For this review, take the finished solid that the model builds, in its own axes (mm). A direction names the side the tool comes from. Coordinates: 2 decimals unless noted, no trailing zeros. Order: outer loops, then holes, each group sorted by start corner. A loop starts at its lowest first (then second) coordinate and runs counter-clockwise, first axis right, second up.
from build123d import *

# Parameters (mm, degrees)
SKETCH1_W                = 82.55
SKETCH1_H                = 53.086
BOSS_EXTRUDE1_DEPTH      = 4.826
CUT_EXTRUDE1_START       = -88.085249325
CUT_EXTRUDE1_OUTLINE_W   = 4.826
CUT_EXTRUDE1_OUTLINE_H   = 4.826
CUT_EXTRUDE1_DEPTH       = 16.51
CUT_EXTRUDE1_START_2     = -55.065249325
CUT_EXTRUDE1_2_OUTLINE_W = 4.826
CUT_EXTRUDE1_2_OUTLINE_H = 4.826
CUT_EXTRUDE1_2_DEPTH     = 16.51
CUT_EXTRUDE1_START_3     = -22.045249325
CUT_EXTRUDE1_3_OUTLINE_W = 4.826
CUT_EXTRUDE1_3_OUTLINE_H = 4.826
CUT_EXTRUDE1_3_DEPTH     = 16.51
SKETCH3_W                = 4.826
SKETCH3_H                = 12.065
CUT_EXTRUDE2_DEPTH       = 97.443575108
SKETCH4_R                = 12.7
CUT_EXTRUDE3_DEPTH       = 97.443575108
SKETCH5_W                = 4.826
SKETCH5_H                = 12.7
CUT_EXTRUDE4_DEPTH       = 97.443575108


# Read off the part's stored shape, not the designer's step: Cut-Extrude1
with BuildPart() as part:
    # Sketch1 → Boss-Extrude1 (new body)
    with BuildSketch(Plane.XY):
        with Locations((-46.810249325, -12.432142782)):
            Rectangle(SKETCH1_W, SKETCH1_H)
    extrude(amount=BOSS_EXTRUDE1_DEPTH)

    # Cut-Extrude1 outline → Cut-Extrude1 (cut)
    with BuildSketch(Plane.YZ.offset(CUT_EXTRUDE1_START)):
        with Locations((11.697857218, 2.413)):
            Rectangle(CUT_EXTRUDE1_OUTLINE_W, CUT_EXTRUDE1_OUTLINE_H)
    extrude(amount=CUT_EXTRUDE1_DEPTH, mode=Mode.SUBTRACT)

    # Cut-Extrude1 2 outline → Cut-Extrude1 2 (cut)
    with BuildSketch(Plane.YZ.offset(CUT_EXTRUDE1_START_2)):
        with Locations((11.697857218, 2.413)):
            Rectangle(CUT_EXTRUDE1_2_OUTLINE_W, CUT_EXTRUDE1_2_OUTLINE_H)
    extrude(amount=CUT_EXTRUDE1_2_DEPTH, mode=Mode.SUBTRACT)

    # Cut-Extrude1 3 outline → Cut-Extrude1 3 (cut)
    with BuildSketch(Plane.YZ.offset(CUT_EXTRUDE1_START_3)):
        with Locations((11.697857218, 2.413)):
            Rectangle(CUT_EXTRUDE1_3_OUTLINE_W, CUT_EXTRUDE1_3_OUTLINE_H)
    extrude(amount=CUT_EXTRUDE1_3_DEPTH, mode=Mode.SUBTRACT)

    # Sketch3 → Cut-Extrude2 (cut, through all)
    with BuildSketch(Plane.XY.offset(4.826)):
        with Locations((-85.672249325, -32.942642782)):
            Rectangle(SKETCH3_W, SKETCH3_H)
        with Locations((-85.672249325, -8.812642782)):
            Rectangle(SKETCH3_W, SKETCH3_H)
        with Locations((-7.948249325, -32.942642782)):
            Rectangle(SKETCH3_W, SKETCH3_H)
        with Locations((-7.948249325, -8.812642782)):
            Rectangle(SKETCH3_W, SKETCH3_H)
    extrude(amount=-CUT_EXTRUDE2_DEPTH, mode=Mode.SUBTRACT)

    # Sketch4 → Cut-Extrude3 (cut, through all)
    with BuildSketch(Plane.XY.offset(4.826)):
        with Locations((-46.810249325, -14.845142782)):
            Circle(SKETCH4_R)
    extrude(amount=-CUT_EXTRUDE3_DEPTH, mode=Mode.SUBTRACT)

    # Sketch5 → Cut-Extrude4 (cut, through all)
    with BuildSketch(Plane.XY.offset(4.826)):
        with Locations((-74.496249325, -9.765142782)):
            Rectangle(SKETCH5_W, SKETCH5_H)
    extrude(amount=-CUT_EXTRUDE4_DEPTH, mode=Mode.SUBTRACT)


solid = part.part
1. Machinability: for faces 1 (the face through (-14, 9.285, 2)), 2 (the face through (-47, 9.285, 2)), 3 (the face through (-75, -3.415, 2)), which of the approach directions +Z, -Z, +X, -X, +Y, -Y give a long, thin tool a straight path to every point of the face, cutting with its end or side? Answer none if there is none.
Answer below:
face 1: +Z, -Z, +X, +Y
face 2: +Z, -Z, +Y
face 3: +Z, -Z
2. Take a section at B-B, the plane y = -9. Give the boundary of the cut face in (x, z).
Answer below:
outline: (-83.26, 0) - (-76.91, 0) - (-76.91, 4.83) - (-83.26, 4.83) - close; (-72.08, 0) - (-58.09, 0) - (-58.09, 4.83) - (-72.08, 4.83) - close; (-35.54, 0) - (-10.36, 0) - (-10.36, 4.83) - (-35.54, 4.83) - close
3. Take a section at C-C, the plane y = -26. Give the boundary of the cut face in (x, z).
Answer below:
outline: (-88.09, 0) - (-52.88, 0) - (-52.88, 4.83) - (-88.09, 4.83) - close; (-40.74, 0) - (-5.54, 0) - (-5.54, 4.83) - (-40.74, 4.83) - close
4. To check wall thickness, follow L1, parallel to Y at x = -14, z = 0.2; L2, parallel to X at y = -13, z = 1.65 (1 decimal); L3, parallel to Y at x = -45, z = 0.4. State the ranges of each line that lie inside material, in increasing order.
Answer below:
L1: y = -38.98 to 9.28
L2: x = -83.3 to -76.9, -72.1 to -59.4, -34.2 to -10.4
L3: y = -38.98 to -27.42, -2.27 to 9.28
5. Take a section at D-D, the plane x = -53.5. Give the boundary of the cut face in (y, z).
Answer below:
outline: (-38.98, 0) - (-25.64, 0) - (-25.64, 4.83) - (-38.98, 4.83) - close; (-4.05, 0) - (9.28, 0) - (9.28, 4.83) - (-4.05, 4.83) - close
6. Clearance check with flat-ended pins moving along their axes: pin 1 Ø1.4 at (y, z) = (-12.5, 3) entering from -X; pin 2 Ø1.4 at (y, z) = (-8.5, 3) entering from +X; pin 3 Ø2.5 at (y, z) = (12, 1.5) entering from +X. State where each tip first meets the part, or that it passes through.
Answer below:
pin 1: stops at x = -83.26
pin 2: stops at x = -10.36
pin 3: stops at x = -22.05
7. Take a section at A-A, the plane z = 2.4. Give the number of separate pieces and of enclosed holes in the cut face, plus the area to 3 significant figures.
Answer below:
separate pieces: 1
enclosed holes: 2
area: 3,340 mm2
8. The part is to be moulded in two halves that separate along Y. For faces 4 (the face through (-86, -14.845, 2)), 5 (the face through (-86, -26.91, 2)), 6 (the face through (-71.575, 12, 2)), say which applies: +Y half, -Y half, draft (parallel to the pull), parting line (faces both ways), or undercut.
Answer below:
face 4: undercut
face 5: -Y half
face 6: draft
